Design review of the part built by this model. Coordinates are the model's own, in mm. A direction names the side the tool comes from. Give positions to 0.01 mm unless a question says otherwise; leave off trailing zeros. Loops run counter-clockwise (first coordinate to the right, second up) from the corner with the lowest first, then second, coordinate; pieces in that order, holes last. Notation, with made-up numbers: M 63.25,82 L 119.25,82 A20 ccw 119.25,113 Z; hole C 6,5 d8. An arc over 180 degrees is marked long. Answer as CSV lines item,"result".
```python
from build123d import *

# Parameters (mm, degrees)
F0_R     = 3.2639
F1_DEPTH = 50.8
F2_R     = 6.35
F2_R_2   = 3.2639
F3_DEPTH = 5.08
F5_DEPTH = 3.81


# Not quite as in the source:
# - a fillet or chamfer that OpenCascade refuses, or shapes differently, is made with other operations: its cross-section is extruded or revolved along the edge and cut away or added


with BuildPart() as f1:
    # F0 (on Front) → F1 (new body)
    with BuildSketch(Plane.XZ):
        Circle(F0_R)
    extrude(amount=F1_DEPTH)

    # F2 (on face) → F3 (join)
    with BuildSketch(Plane(origin=(0, 0, 0), x_dir=(-1, 0, 0), z_dir=(0, 1, 0))):
        Circle(F2_R)
        Circle(F2_R_2, mode=Mode.SUBTRACT)
        Circle(F2_R_2)
    extrude(amount=F3_DEPTH)

    # F4 (on face) → F5 (cut)
    with BuildSketch(Plane(origin=(0, 5.08, 0), x_dir=(-1, 0, 0), z_dir=(0, 1, 0))):
        Polygon((-1.9368684152, 3.1454528216), (-3.6924762575, -0.1046508405), (-1.7556078423, -3.2501036622), (1.9368684152, -3.1454528216), (3.6924762575, 0.1046508405), (1.7556078423, 3.2501036622), align=None)
    extrude(amount=-F5_DEPTH, mode=Mode.SUBTRACT)

    # F6: fillet of radius 3.81 on 1 edges, made by hand

    # F6_s1 → F6_t2 (revolve, cut)
    with BuildSketch(Plane.XY):
        with BuildLine():
            ThreePointArc((-6.35, 1.27), (-5.2340768363, 3.9640768363), (-2.54, 5.08))
            Line((-2.54, 5.08), (-6.35, 5.08))
            Line((-6.35, 5.08), (-6.35, 1.27))
        make_face()
    revolve(axis=Axis((0, 5.08, 0), (0, 1, 0)), mode=Mode.SUBTRACT)


solid = f1.part
```
1. For P1, Ø6, axis at x = 4, y = -25, coming from the -Z side; P2, Ø6, axis at y = -44, z = 5, coming from the -X side; P3, Ø4, axis at y = -11.5, z = -2.5, coming from the +X side, all flat-tipped, find the tip position at first contact; note any pin that passes through.
Answer block:
P1,"z = -3.11"
P2,"x = -2.58"
P3,"x = 3.23"
2. We need section A-A, the plane y = -19.5. Write out the cut boundary in (x, z), plus the area to 3 significant figures.
Answer block:
outline,"C 0,0 d6.53"
area,"33.5 mm²"
3. To check wall thickness, follow L1, parallel to Y at x = -2.5, z = 0; L2, parallel to Y at x = -2, z = 5.5; L3, parallel to Z at x = 1, y = -11.5. State the ranges of each line that lie inside material, in increasing order. Write a range as [from, to].
Answer block:
L1,"[-50.8, 1.27]"
L2,"[0, 3.15]"
L3,"[-3.11, 3.11]"
4. For faces 1 (the cylindrical face through (-0.708, -25.044, -3.186)), 2 (the flat face through (-2.802, 3.173, -1.543)), 3 (the flat face through (0, -50.8, 0)), list the 3-axis set-ups (+Z, -Z, +X, -X, +Y, -Y) from which the entire face can be reached by the end or side of a thin tool; tool diameter is ignored.
Answer block:
face 1,"-Y"
face 2,"+Y"
face 3,"+Z, -Z, +X, -X, -Y"
5. The part is to be moulded in two halves that separate along Z. For faces 4 (the flat face through (-2.738, 3.173, 1.655)), 5 (the flat face through (3, 0, 2)), 6 (the cylindrical face through (1.38, 0.63, -6.2)), say which applies: pulls with the +Z half, pulls with the -Z half, needs draft (parallel to the pull), parting line crosses it, or undercut.
Answer block:
face 4,"undercut"
face 5,"needs draft"
face 6,"parting line crosses it"
